Check sheet for the drawn part. Datum: minimum x, y, z corner. Units: mm. Give positions to 0.01 mm unless a question says otherwise; leave off trailing zeros. Loops run counter-clockwise (first coordinate to the right, second up) from the corner with the lowest first, then second, coordinate; pieces in that order, holes last. Notation, with made-up numbers: (28.5, -14) - (67.5, -14) arc R18 cw to (67.5, 17) - close; hole circle Ø9 at (-31, 31). An arc over 180 degrees is marked (long way). Use a Markdown table: item, result. Add a question column.
1. Material ranges on L1, parallel to X at y = 0.9, z = 6.35; L2, parallel to X at y = 2, z = 7.25 (1 decimal); L3, parallel to X at y = 2.6, z = 4.25, recorded low to high.
2. Cross-section at D-D on y = 1.55. Enter the section's corners in (x, z), and give its area (3 significant figures).
3. Cross-section at A-A on x = 6.35. Enter the section's corners in (y, z) (1 decimal).
4. Depth check by flat-ended pin: P1, Ø1.5, axis at x = 2.5, y = 2.5, coming from the +Z side; P2, Ø1, axis at x = 3, y = 1, coming from the +Z side (1 decimal); P3, Ø1.4, axis at x = 6.35, z = 6.35, coming from the -Y side; P4, Ø1.5, axis at x = 3, y = 2.5, coming from the +Z side. Enter the tip coordinate at first touch or a pass-through.
5. Cross-section at C-C on y = 2.85. Enter the section's corners in (x, z).
6. Cross-section at B-B on z = 6.35. Enter the section's corners in (x, y) (1 decimal).
7. Draft check along Z on the marked faces 1, 2 and 3. Enter one of: pulls with the +Z half, pulls with the -Z half, needs draft (parallel to the pull), parting line crosses it, or undercut.
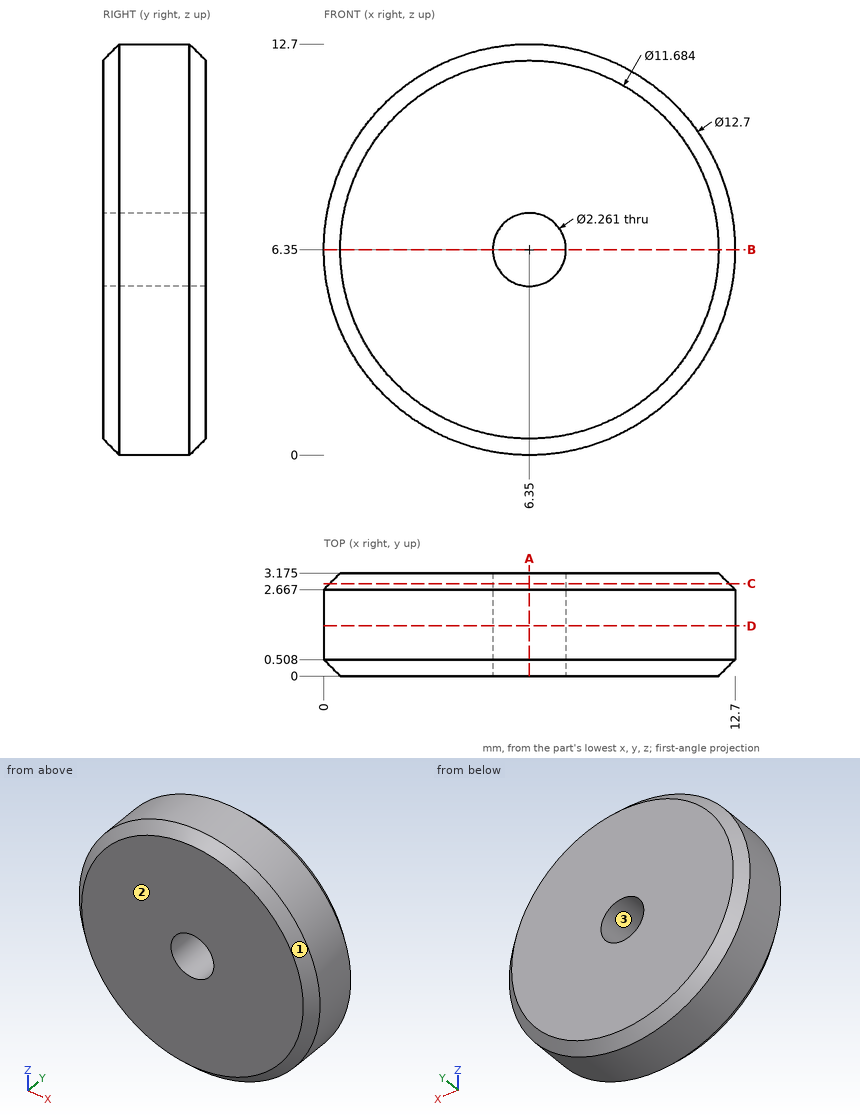
Values found:
| question | item | result |
|---|---|---|
| 1 | L1 | x = 0 to 5.22, 7.48 to 12.7 |
| 1 | L2 | x = 0.1 to 5.7, 7 to 12.6 |
| 1 | L3 | x = 0.36 to 12.34 |
| 2 | outline | circle Ø12.7 at (6.35, 6.35); hole circle Ø2.26 at (6.35, 6.35) |
| 2 | area | 123 mm2 |
| 3 | outline | (0, 0.5) - (0.5, 0) - (2.7, 0) - (3.2, 0.5) - (3.2, 5.2) - (0, 5.2) - close; (0, 7.5) - (3.2, 7.5) - (3.2, 12.2) - (2.7, 12.7) - (0.5, 12.7) - (0, 12.2) - close |
| 4 | P1 | stops at z = 11.89 |
| 4 | P2 | stops at z = 12 |
| 4 | P3 | passes through |
| 4 | P4 | stops at z = 12.14 |
| 5 | outline | circle Ø12.33 at (6.35, 6.35); hole circle Ø2.26 at (6.35, 6.35) |
| 6 | outline | (0, 0.5) - (0.5, 0) - (5.2, 0) - (5.2, 3.2) - (0.5, 3.2) - (0, 2.7) - close; (7.5, 0) - (12.2, 0) - (12.7, 0.5) - (12.7, 2.7) - (12.2, 3.2) - (7.5, 3.2) - close |
| 7 | face 1 | parting line crosses it |
| 7 | face 2 | needs draft |
| 7 | face 3 | undercut |
